Design review of the part shown in the three views and the two pictorial views. Dimensions are in mm from the part's minimum x, y and z. A direction names the side the tool comes from. Coordinates: 2 decimals unless noted, no trailing zeros. Loops run counter-clockwise (first coordinate to the right, second up) from the corner with the lowest first, then second, coordinate; pieces in that order, holes last. Notation, with made-up numbers: (51.25, 41.5) -> (68.25, 41.5) arc R27 ccw to (68.25, 72.5) -> close; hole circle Ø9 at (-35.75, -13). An arc over 180 degrees is marked (long way). Answer in a Markdown table with one row per item.
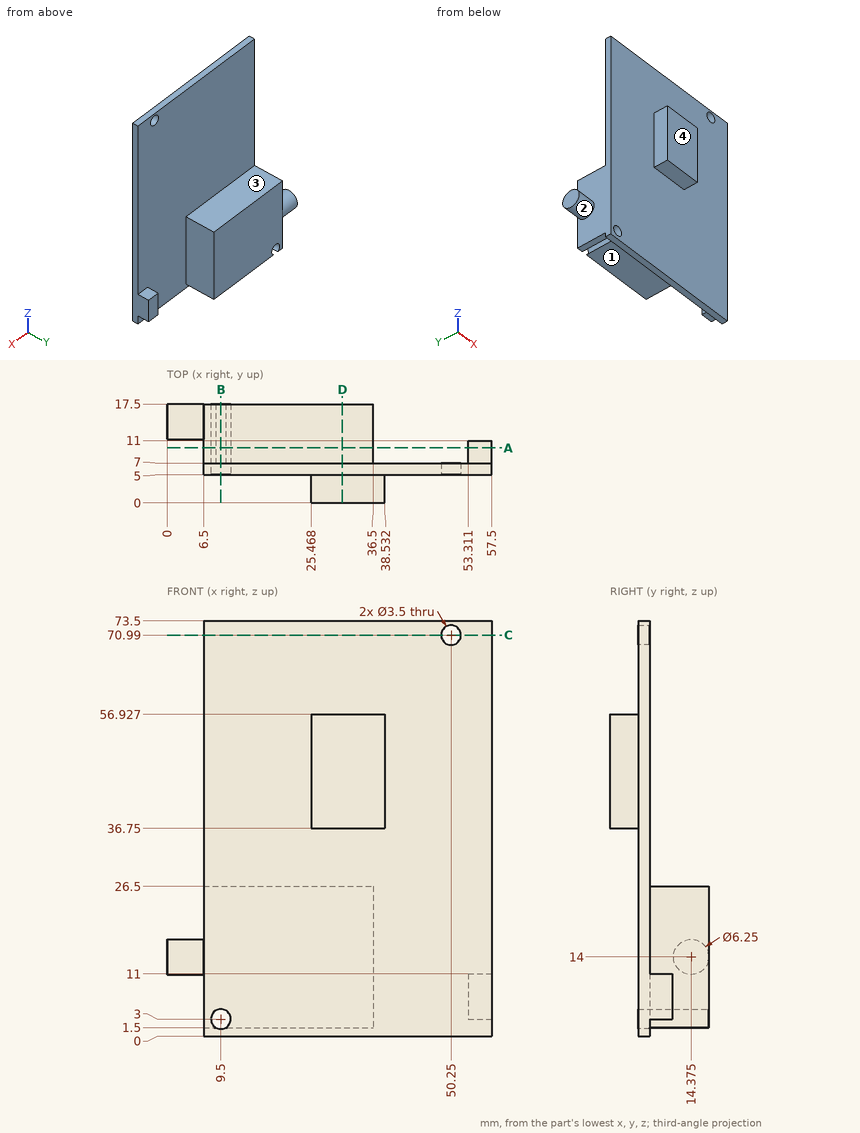
(1) Tool access review of the marked faces 1, 2, 3 and 4: name each direction out of +Z, -Z, +X, -X, +Y, -Y from which nothing blocks a thin tool from reaching the whole face with its end or side.
Evaluation:
| item | result |
|---|---|
| face 1 | -Z, +X, -X, +Y |
| face 2 | -X |
| face 3 | +Z, +X, -X, +Y |
| face 4 | +Z, -Z, +X, -X, -Y |
(2) Take a section at C-C on z = 70.99. Give the boundary of the cut face in (x, y).
Evaluation:
| item | result |
|---|---|
| outline | (6.5, 5) -> (48.5, 5) -> (48.5, 7) -> (6.5, 7) -> close; (52, 5) -> (57.5, 5) -> (57.5, 7) -> (52, 7) -> close |
(3) To check wall thickness, follow probe 1 along X at (y, z) = (13, 3); probe 2 along Z at (x, y) = (50.25, 6.05); probe 3 along X at (y, z) = (5.4, 70.99). State the ranges of each line that lie inside material, in increasing order.
Evaluation:
| item | result |
|---|---|
| probe 1 | x = 6.5 to 7.75, 11.25 to 36.5 |
| probe 2 | z = 0 to 69.24, 72.74 to 73.5 |
| probe 3 | x = 6.5 to 48.5, 52 to 57.5 |
(4) Take a section at B-B on x = 9.5. Give the boundary of the cut face in (y, z).
Evaluation:
| item | result |
|---|---|
| outline | (5, 0) -> (7, 0) -> (7, 1.25) -> (5, 1.25) -> close; (5, 4.75) -> (17.5, 4.75) -> (17.5, 26.5) -> (7, 26.5) -> (7, 73.5) -> (5, 73.5) -> close |
(5) Take a section at A-A on y = 9.75. Give the boundary of the cut face in (x, z), and give its area (3 significant figures).
Evaluation:
| item | result |
|---|---|
| outline | (6.5, 1.5) -> (8.6, 1.5) arc R1.75 cw (long way) to (10.4, 1.5) -> (36.5, 1.5) -> (36.5, 26.5) -> (6.5, 26.5) -> close; (53.31, 3) -> (57.5, 3) -> (57.5, 11) -> (53.31, 11) -> close |
| area | 774 mm² |
(6) Take a section at D-D on x = 31. Give the boundary of the cut face in (y, z).
Evaluation:
| item | result |
|---|---|
| outline | (0, 36.75) -> (5, 36.75) -> (5, 0) -> (7, 0) -> (7, 1.5) -> (17.5, 1.5) -> (17.5, 26.5) -> (7, 26.5) -> (7, 73.5) -> (5, 73.5) -> (5, 56.93) -> (0, 56.93) -> close |
(7) For pin 1 (8 mm diameter, centred on x = 46, z = 29, fed in from +Y); pin 2 (8 mm diameter, centred on y = 10, z = 15.5, fed in from -X); pin 3 (1.2 mm diameter, centred on x = 55, y = 9.5, fed in from +Z); pin 4 (6 mm diameter, centred on x = 11.5, y = 15, fed in from -Z), all flat-tipped, find the tip position at first contact; note any pin that passes through.
Evaluation:
| item | result |
|---|---|
| pin 1 | stops at y = 7 |
| pin 2 | stops at x = 0 |
| pin 3 | stops at z = 11 |
| pin 4 | stops at z = 1.5 |
